Verification items for the finished model (mm, model axes). A direction names the side the tool comes from. Coordinates: 2 decimals unless noted, no trailing zeros. Write each loop counter-clockwise with the first axis right and the second up, starting at its lowest first coordinate (ties: lowest second). Pieces come first, ordered by that corner, then holes. Notation, with made-up numbers: (-32, -9) -> (-12, -9) arc R14 cw to (-12, 3) -> close; hole circle Ø6 at (65.25, -7). An arc over 180 degrees is marked (long way). Answer in a Markdown table with one row per item.
```python
from build123d import *

# Parameters (mm, degrees)
BOSS_EXTRUDE1_DEPTH      = 2
SKETCH2_R                = 3
SKETCH2_W                = 2
SKETCH2_H                = 6
SKETCH2_W_2              = 19.404886506
SKETCH2_H_2              = 107.587058951
SKETCH2_W_3              = 12
SKETCH2_H_3              = 62.119371688
SKETCH2_W_4              = 6
SKETCH2_H_4              = 2
SKETCH2_W_5              = 5
SKETCH2_W_6              = 87.5481705
SKETCH2_H_5              = 43.571241204
SKETCH2_W_7              = 79
SKETCH2_H_6              = 60.456746524
CUT_EXTRUDE1_DEPTH       = 10
BOSS_EXTRUDE2_DEPTH      = 10
BOSS_EXTRUDE2_DEPTH_BACK = 2
FILLET1_R                = 2
CUT_EXTRUDE2_DEPTH       = 10
CUT_EXTRUDE2_DEPTH_BACK  = 10
SKETCH5_R                = 2.5
SKETCH5_R_2              = 2
CUT_EXTRUDE3_DEPTH       = 10


with BuildPart() as part:
    # Sketch1 → Boss-Extrude1 (new body)
    with BuildSketch(Plane.XY):
        Polygon((-10.904784398, -69.72039113), (-10.904784398, 69.72039113), (167.095215602, 120.741927431), (167.095215602, -120.741927431), align=None)
    extrude(amount=BOSS_EXTRUDE1_DEPTH)

    # Sketch2 → Cut-Extrude1 (cut)
    with BuildSketch(Plane.XY.offset(2)):
        with Locations((47.563666615, 2.7699494)):
            Circle(SKETCH2_R)
        with Locations((47.563666615, 73.7699494)):
            Circle(SKETCH2_R)
        with Locations((30.687477401, 41.636914827)):
            Rectangle(SKETCH2_W, SKETCH2_H)
        with Locations((30.687477401, -37.025532441)):
            Rectangle(SKETCH2_W, SKETCH2_H)
        with Locations((-4.312522599, 41.636914827)):
            Rectangle(SKETCH2_W, SKETCH2_H)
        with Locations((-4.312522599, -37.025532441)):
            Rectangle(SKETCH2_W, SKETCH2_H)
        with Locations((13.187477401, 2.305691192)):
            Rectangle(SKETCH2_W_2, SKETCH2_H_2)
        with Locations((46.32953553, -40.519587511)):
            Rectangle(SKETCH2_W_3, SKETCH2_H_3)
        with Locations((78.467345618, -87.370243237)):
            Rectangle(SKETCH2_W_4, SKETCH2_H_4)
        with Locations((78.467345618, -12.370243237)):
            Rectangle(SKETCH2_W_4, SKETCH2_H_4)
        with Locations((151.467345618, -87.370243237)):
            Rectangle(SKETCH2_W_4, SKETCH2_H_4)
        with Locations((151.467345618, -12.370243237)):
            Rectangle(SKETCH2_W_4, SKETCH2_H_4)
        with Locations((84.496263797, 1.389968406)):
            Rectangle(SKETCH2_W_5, SKETCH2_H_4)
        with Locations((84.496263797, 88.389968406)):
            Rectangle(SKETCH2_W_5, SKETCH2_H_4)
        with Locations((144.496263797, 88.389968406)):
            Rectangle(SKETCH2_W_5, SKETCH2_H_4)
        with Locations((144.496263797, 1.389968406)):
            Rectangle(SKETCH2_W_5, SKETCH2_H_4)
        with Locations((117.693260368, -51.579694355)):
            Rectangle(SKETCH2_W_6, SKETCH2_H_5)
        with Locations((114.967345618, 45.962282478)):
            Rectangle(SKETCH2_W_7, SKETCH2_H_6)
    extrude(amount=-CUT_EXTRUDE1_DEPTH, mode=Mode.SUBTRACT)

    # Sketch3 → Boss-Extrude2 (add, two sides)
    with BuildSketch(Plane(origin=(0, 0, 0), x_dir=(-1, 0, 0), z_dir=(0, 0, -1))) as boss_extrude2_sk:
        Polygon((10.904784398, -69.72039113), (-167.095215602, -120.741927431), (-167.095215602, -122.741927431), (10.904784398, -71.72039113), align=None)
        Polygon((-167.095215602, 120.741927431), (-167.095215602, 122.741927431), (10.904784398, 71.72039113), (10.904784398, 69.72039113), align=None)
    extrude(amount=BOSS_EXTRUDE2_DEPTH)
    extrude(boss_extrude2_sk.sketch, amount=-BOSS_EXTRUDE2_DEPTH_BACK)

    # Fillet1
    fillet1_edges = [part.edges().sort_by_distance(p)[0] for p in [
        (78.095215602, -97.231159281, 2),
        (78.095215602, 97.231159281, 2),
        (78.095215602, -95.231159281, 0),
        (78.095215602, 95.231159281, 0),
    ]]
    fillet(fillet1_edges, radius=FILLET1_R)

    # Sketch4 → Cut-Extrude2 (cut, two sides)
    with BuildSketch(Plane(origin=(0, 0, 0), x_dir=(-1, 0, 0), z_dir=(0, 0, -1))) as cut_extrude2_sk:
        Polygon((-29.095215602, 79.105365308), (-127.095215602, 107.195874059), (-129.724486678, 107.949522652), (-128.643652311, 111.720254216), (-128.09256865, 113.642832381), (-127.51525552, 115.656917896), (-124.890880959, 114.886186717), (-26.890880959, 86.105365308), align=None)
        Polygon((-127.095215602, -107.195874059), (-129.724486678, -107.949522652), (-128.643652311, -111.720254216), (-128.09256865, -113.642832381), (-127.51525552, -115.656917896), (-124.890880959, -114.886186717), (-26.890880959, -86.105365308), (-29.095215602, -79.105365308), align=None)
    extrude(amount=CUT_EXTRUDE2_DEPTH, mode=Mode.SUBTRACT)
    extrude(cut_extrude2_sk.sketch, amount=-CUT_EXTRUDE2_DEPTH_BACK, mode=Mode.SUBTRACT)

    # Sketch5 → Cut-Extrude3 (cut)
    with BuildSketch(Plane(origin=(-19.29514045, -67.315397557, 0), x_dir=(0.961289082, -0.27554183, 0), z_dir=(0.27554183, 0.961289082, 0))):
        with Locations((173.896258148, 6)):
            Circle(SKETCH5_R)
        with Locations((28.728234, 6)):
            Circle(SKETCH5_R_2)
    cut_extrude3 = extrude(amount=-CUT_EXTRUDE3_DEPTH, mode=Mode.SUBTRACT)

    # Mirror1: Cut-Extrude3 across plane
    add(cut_extrude3.mirror(Plane.ZX), mode=Mode.SUBTRACT)


solid = part.part
```
1. Thickness scan on line 1 (X direction, y = 47, z = 1); line 2 (Z direction, x = 100, y = 6.5); line 3 (Y direction, x = 136, z = -4). Record the ranges inside material, lowest first. Write a range as from..to.
Geometry says:
| item | result |
|---|---|
| line 1 | -10.9..3.49, 22.89..75.47, 154.47..167.1 |
| line 2 | 0..2 |
| line 3 | -113.83..-111.83, 111.83..113.83 |
2. Section check D-D, the plane x = 132.5. State how many separate pieces and enclosed holes the cut face has, plus the area to 3 significant figures.
Geometry says:
| item | result |
|---|---|
| separate pieces | 3 |
| enclosed holes | 0 |
| area | 283 mm^2 |
3. Depth check by flat-ended pin: P1, Ø1, axis at x = 80, z = 1, coming from the -Y side; P2, Ø2, axis at x = 30.5, z = 0.5, coming from the +Y side; P3, Ø5.5, axis at x = 47.56, y = 73.77, coming from the -Z side; P4, Ø1.6, axis at x = 10, z = 1.5, coming from the -Y side. Enter the tip coordinate at first touch or a pass-through.
Geometry says:
| item | result |
|---|---|
| P1 | y = -93.84 |
| P2 | y = 79.79 |
| P3 | through |
| P4 | y = -77.65 |
4. Section check B-B, the plane y = -58.5. Record the boundary of the cut face in (x, z).
Geometry says:
| item | result |
|---|---|
| outline | (-10.9, 0) -> (40.33, 0) -> (40.33, 2) -> (-10.9, 2) -> close; (52.33, 0) -> (73.92, 0) -> (73.92, 2) -> (52.33, 2) -> close; (161.47, 0) -> (167.1, 0) -> (167.1, 2) -> (161.47, 2) -> close |
5. Mould release check, pull along X, two halves, no side actions. Record for faces 3 (the flat face through (148.14, 117.31, -2.85)), 4 (the flat face through (8.52, -75.29, -3.28)), 5 (the cylindrical face through (44.567, 2.902, 1.014)): released by +X, released by -X, zero draft, split by the parting line, or undercut.
Geometry says:
| item | result |
|---|---|
| face 3 | released by -X |
| face 4 | released by +X |
| face 5 | undercut |
6. Section check C-C, the plane x = 102.5. Record the boundary of the cut face in (y, z), plus the area to 3 significant figures.
Geometry says:
| item | result |
|---|---|
| outline | (-100.15, 0) -> (-73.37, 0) -> (-73.37, 2) -> (-100.15, 2) -> close; (-29.79, 0) -> (15.73, 0) -> (15.73, 2) -> (-29.79, 2) -> close; (76.19, 0) -> (100.15, 0) -> (100.15, 2) -> (76.19, 2) -> close |
| area | 193 mm^2 |
7. Section check A-A, the plane y = 59. Record the boundary of the cut face in (x, z).
Geometry says:
| item | result |
|---|---|
| outline | (-10.9, 0) -> (75.47, 0) -> (75.47, 2) -> (-10.9, 2) -> close; (154.47, 0) -> (167.1, 0) -> (167.1, 2) -> (154.47, 2) -> close |
8. Tool access check on faces 1 (the flat face through (8.52, 75.29, -3.28)), 2 (the flat face through (148, -116, -10)). Record the directions out of +Z, -Z, +X, -X, +Y, -Y that give a thin tool (end or side, any length) a straight path to the whole face; none if there is none.
Geometry says:
| item | result |
|---|---|
| face 1 | -Z, +X |
| face 2 | -Z, +X, -X, +Y, -Y |
